Can you work these out from the model? Positions are in its coordinate system, mm. Round coordinates to 2 decimals unless told otherwise and drop trailing zeros. Order: outer loops, then holes, each group sorted by start corner. A loop starts at its lowest first (then second) coordinate and runs counter-clockwise, first axis right, second up. Notation, with made-up numbers: M -40,42.25 L 8,42.25 A19 ccw 8,62.25 Z; hole C 10,53 d8. An arc over 180 degrees is marked long. Answer as CSV lines item,"result". Start each with the question number.
from build123d import *

# Parameters (mm, degrees)
F0_R     = 17.5
F1_DEPTH = 1
F2_R     = 17.5
F2_R_2   = 2.5
F2_R_3   = 2.45
F3_DEPTH = 1.75


with BuildPart() as f1:
    # F0 (on Top) → F1 (new body)
    with BuildSketch(Plane.XY):
        Circle(F0_R)
    extrude(amount=F1_DEPTH)

    # F2 (on face) → F3 (join)
    with BuildSketch(Plane.XY.offset(1)):
        Circle(F2_R)
        with Locations((-9.477707, -6.945183)):
            Circle(F2_R_2, mode=Mode.SUBTRACT)
        with Locations((1.275852, -11.680527)):
            Circle(F2_R_2, mode=Mode.SUBTRACT)
        with Locations((10.753559, -4.735343)):
            Circle(F2_R_2, mode=Mode.SUBTRACT)
        with Locations((-10.753559, 4.735343)):
            Circle(F2_R_3, mode=Mode.SUBTRACT)
        with Locations((-1.275852, 11.680527)):
            Circle(F2_R_2, mode=Mode.SUBTRACT)
        with Locations((9.477707, 6.945183)):
            Circle(F2_R_2, mode=Mode.SUBTRACT)
    extrude(amount=F3_DEPTH)


solid = f1.part
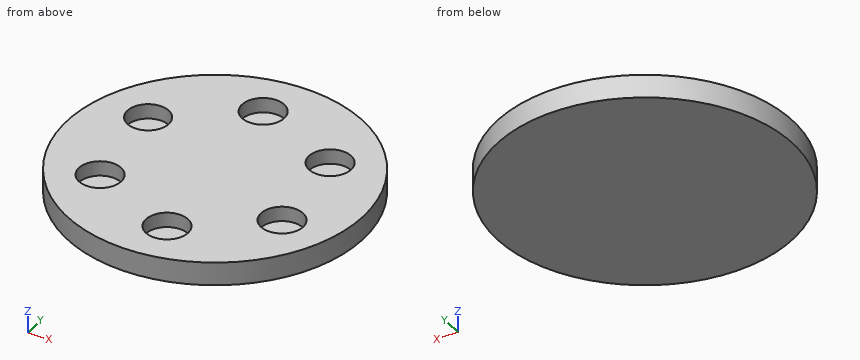
(1) I want a section at A-A on x = 0. Write out the boundary of the cut face in (y, z).
(2) I want a section at D-D on x = -9. Write out the boundary of the cut face in (y, z).
(3) I'm going to push a flat-ended pin straight in: P1, Ø3, axis at x = -1.28, y = 11.68, coming from the +Z side. Where does the tip first touch, or does it pass through?
(4) I want a section at C-C on y = -3. Write out the boundary of the cut face in (x, z).
(5) If I drill on line 1 along Y through (x, z) = (0.5, 2.55); line 2 along X through (y, z) = (-5, 1.8); line 3 along X through (y, z) = (4, 2.1), over which ranges is the centre line in solid material (lowest first)?
(6) I want a section at B-B on z = 1.4. Write out the boundary of the cut face in (x, y).
From the geometry:
1,outline,"M -17.5,0 L 17.5,0 L 17.5,2.75 L 13.83,2.75 L 13.83,1 L 9.53,1 L 9.53,2.75 L -9.53,2.75 L -9.53,1 L -13.83,1 L -13.83,2.75 L -17.5,2.75 Z"
2,outline,"M -15.01,0 L 15.01,0 L 15.01,2.75 L 6.45,2.75 L 6.45,1 L 3.02,1 L 3.02,2.75 L -4.49,2.75 L -4.49,1 L -9.4,1 L -9.4,2.75 L -15.01,2.75 Z"
3,P1,"z = 1"
4,outline,"M -17.24,0 L 17.24,0 L 17.24,2.75 L 12.55,2.75 L 12.55,1 L 8.95,1 L 8.95,2.75 L -17.24,2.75 Z"
5,line 1,"-17.49 to -14.06, -9.3 to 9.92, 13.44 to 17.49"
5,line 2,"-16.77 to -11.05, -7.91 to 8.27, 13.24 to 16.77"
5,line 3,"-17.04 to -13.09, -8.42 to 17.04"
6,outline,"C 0,0 d35; hole C -10.75,4.74 d4.9; hole C -9.48,-6.95 d5; hole C -1.28,11.68 d5; hole C 1.28,-11.68 d5; hole C 9.48,6.95 d5; hole C 10.75,-4.74 d5"
